```python
from build123d import *

# Parameters (mm, degrees)
SKETCH1_R          = 19
EXTRUDE13_DEPTH    = 63
EXTRUDE15_DEPTH    = 17
SKETCH2_R          = 19.5
EXTRUDE18_DEPTH    = 24
SKETCH2_6_R        = 19.5
CUT_EXTRUDE1_DEPTH = 14.38
SKETCH7_W          = 85
SKETCH7_H          = 47.220330203
EXTRUDE21_DEPTH    = 27.6


with BuildPart() as part:
    # Sketch1 → Extrude13 (new body)
    with BuildSketch(Plane.XY):
        with Locations((9.080174701, 18.537445764)):
            Circle(SKETCH1_R)
        with BuildLine():
            ThreePointArc((-0.037230939, 16.976864339), (-0.16055511, 18.123425772), (-0.140259902, 19.276421901))
            ThreePointArc((-0.140259902, 19.276421901), (-0.057438126, 18.128045807), (-0.037230939, 16.976864339))
        make_face(mode=Mode.SUBTRACT)
    extrude(amount=-EXTRUDE13_DEPTH)

    # Sketch1<17> → Extrude15 (add)
    with BuildSketch(Plane.XY):
        with BuildLine():
            ThreePointArc((-0.140259902, 19.276421901), (-0.057438126, 18.128045807), (-0.037230939, 16.976864339))
            ThreePointArc((-0.037230939, 16.976864339), (18.320904513, 18.951465757), (-0.140259902, 19.276421901))
        make_face()
    extrude(amount=EXTRUDE15_DEPTH)



with BuildPart() as body_2:
    # Sketch2 → Extrude18 (new body)
    with BuildSketch(Plane.XY):
        with Locations((-45.03001877, 0)):
            Circle(SKETCH2_R)
    extrude(amount=EXTRUDE18_DEPTH)

    # Sketch2<6> → Cut-Extrude1 (cut)
    with BuildSketch(Plane.XY):
        with Locations((-45.03001877, 0)):
            Circle(SKETCH2_6_R)
    extrude(amount=CUT_EXTRUDE1_DEPTH, mode=Mode.SUBTRACT)


with BuildPart() as part_1:
    add(part.part)

    add(body_2.part)  # Extrude21 merges body 2
    # Sketch7 → Extrude21 (add)
    with BuildSketch(Plane.XY):
        with Locations((-20.041402411, 16.059391911)):
            Rectangle(SKETCH7_W, SKETCH7_H)
    extrude(amount=EXTRUDE21_DEPTH)


solid = part_1.part
```
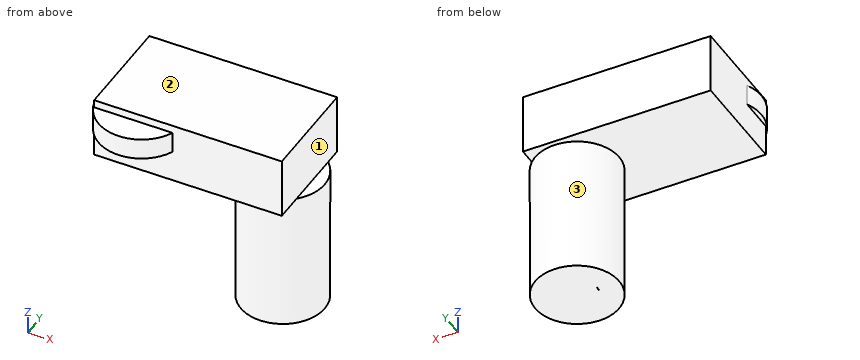
Here's how the part is built. I have some questions about the finished solid (model axes, mm). Face numbers are marked on the shaded views. A direction names the side the tool comes from. Give positions to 0.01 mm unless a question says otherwise; leave off trailing zeros. Write each loop counter-clockwise with the first axis right and the second up, starting at its lowest first coordinate (ties: lowest second). Pieces come first, ordered by that corner, then holes.
(1) Imagine slicing it at A-A, the plane x = 3. Write out the boundary of the cut face in (y, z).
Output values:
outline: (-7.55, 0) - (0.54, 0) - (0.54, -63) - (36.54, -63) - (36.54, 0) - (39.67, 0) - (39.67, 27.6) - (-7.55, 27.6) - close
(2) Will these pins go through, and if not, where does the flat tip stop? pin 1 (23.5 mm diameter, centred on x = -36.5, y = 9, fed in from -Z); pin 2 (10 mm diameter, centred on y = 18, z = 1, fed in from -X); pin 3 (22 mm diameter, centred on y = 16, z = 7.5, fed in from -X).
Output values:
pin 1: stops at z = 0
pin 2: stops at x = -62.54
pin 3: stops at x = -63.06
(3) On a 3-axis mill with a long thin cutter (end or side, diameter ignored), from which of +Z, -Z, +X, -X, +Y, -Y can I reach the whole of each face in a straight line? I mean the marked faces 1, 2 and 3. Say none if no direction works.
Output values:
face 1: +Z, +X, +Y, -Y
face 2: +Z, +X, -X, +Y, -Y
face 3: -Z
(4) Imagine slicing it at C-C, the plane z = -25.5. Write out the boundary of the cut face in (x, y).
Output values:
outline: circle Ø38 at (9.08, 18.54); hole (-0.14, 19.28) arc R9.25 ccw to (-0.04, 16.98) arc R21.15 ccw to start
(5) If I drill on L1, parallel to Z at x = -22.5, y = 8; L2, parallel to Z at x = -58, y = -14; L3, parallel to Y at x = 5.5, z = 2, over which ranges is the centre line in solid material (lowest first)?
Output values:
L1: z = 0 to 27.6
L2: z = 14.38 to 24
L3: y = -7.55 to 39.67
(6) Imagine slicing it at B-B, the plane y = -5.5. Write out the boundary of the cut face in (x, z), and give its area (3 significant figures).
Output values:
outline: (-63.74, 14.38) - (-62.54, 14.38) - (-62.54, 0) - (22.46, 0) - (22.46, 27.6) - (-62.54, 27.6) - (-62.54, 24) - (-63.74, 24) - close
area: 2,360 mm2
